Read the model definition and answer for the solid it produces. Units are mm, in the model's axes. Coordinates: 2 decimals unless noted, no trailing zeros. Order: outer loops, then holes, each group sorted by start corner. A loop starts at its lowest first (then second) coordinate and runs counter-clockwise, first axis right, second up.
from build123d import *

# Parameters (mm, degrees)
SKETCH1_W           = 25
SKETCH1_H           = 14
SKETCH1_R           = 1
BOSS_EXTRUDE1_DEPTH = 5


with BuildPart() as part:
    # Sketch1 → Boss-Extrude1 (new body)
    with BuildSketch(Plane(origin=(0, 0, 0), x_dir=(1, 0, 0), z_dir=(0, 1, 0))):
        Rectangle(SKETCH1_W, SKETCH1_H)
        with Locations(Location((7.5, 0, 0), (0, 0, 270))):
            Circle(SKETCH1_R, mode=Mode.SUBTRACT)
        with Locations(Location((-7.5, 0, 0), (0, 0, 270))):
            Circle(SKETCH1_R, mode=Mode.SUBTRACT)
    extrude(amount=BOSS_EXTRUDE1_DEPTH)

    # Sketch2 → Revolve-Thin1 (revolve)
    with BuildSketch(Plane.XY):
        with BuildLine():
            ThreePointArc((0, -10), (-6, -4), (0, 2))
            Line((0, 2), (0, 1))
            ThreePointArc((0, 1), (-5, -4), (0, -9))
            Line((0, -9), (0, -10))
        make_face()
    revolve(axis=Axis((0, 2, 0), (0, -1, 0)))


solid = part.part
Q1. Straight lines are drawn through the part: L1, parallel to X at y = 2.4, z = 0; L2, parallel to Y at x = -11.5, z = 1; L3, parallel to Z at x = 2.75, y = -5. For each, find the intervals that lie inside material, in ascending order.
Q2. The part is cut by section A-A, the plane z = 0. Determine the outline of the cut face in (x, y).
Q3. Determine the mould class of faces 1 (the cylindrical face through (-6.51, 2.46, -0.13)), 2 (the flat face through (0, 2, 7)), 3 (the flat face through (0, 0, 0)), 4 (the flat face through (12.5, 2, 0)) for opening direction Z: +Z half, -Z half, draft (parallel to the pull), parting line (faces both ways), or undercut.
Q4. The part is cut by section D-D, the plane z = -1.5. Determine the outline of the cut face in (x, y).
Q5. Each of these flat-tipped pins is pushed along its axis until it touches: P1, Ø5, axis at x = 0, y = -3.5, coming from the +Z side; P2, Ø8, axis at y = -2, z = -5.5, coming from the +X side; P3, Ø2, axis at y = -3.5, z = -1.5, coming from the -X side; P4, Ø1.5, axis at x = 8.5, z = 4, coming from the -Y side. Where does it stop, or does it pass through?
Q6. The part is cut by section C-C, the plane y = 0.75. Determine the outline of the cut face in (x, z).
Q7. The part is cut by section B-B, the plane x = -7.5. Determine the outline of the cut face in (y, z), then the cut area to 3 significant figures.
Computed values:
1. L1: x = -12.5 to -8.5, -6.5 to 6.5, 8.5 to 12.5
1. L2: y = 0 to 5
1. L3: z = -5.24 to -4.05, 4.05 to 5.24
2. outline: (-12.5, 0) - (-8.5, 0) - (-8.5, 5) - (-12.5, 5) - close; (-6.5, 0) - (-4.47, 0) arc R6 ccw (long way) to (4.47, 0) - (6.5, 0) - (6.5, 5) - (-6.5, 5) - close; (8.5, 0) - (12.5, 0) - (12.5, 5) - (8.5, 5) - close; hole (-3, 0) arc R5 ccw (long way) to (3, 0) - close
3. face 1: undercut
3. face 2: +Z half
3. face 3: undercut
3. face 4: draft
4. outline: (-12.5, 0) - (-4.21, 0) arc R5.81 ccw (long way) to (4.21, 0) - (12.5, 0) - (12.5, 5) - (-12.5, 5) - close; hole (-2.6, 0) arc R4.77 ccw (long way) to (2.6, 0) - close
5. P1: stops at z = 6
5. P2: stops at x = 12.5
5. P3: stops at x = -5.97
5. P4: stops at y = 0
6. outline: (-12.5, -7) - (12.5, -7) - (12.5, 7) - (-12.5, 7) - close; hole circle Ø2 at (-7.5, 0); hole circle Ø2 at (7.5, 0)
7. outline: (0, -7) - (5, -7) - (5, -1) - (0, -1) - close; (0, 1) - (5, 1) - (5, 7) - (0, 7) - close
7. area: 60.0 mm2
